Input: part model. Units: mm. Frame: model coordinates. Face numbers are marked on the shaded views. A direction names the side the tool comes from. Give positions to 0.01 mm unless a question says otherwise; leave off trailing zeros. Loops run counter-clockwise (first coordinate to the right, second up) from the corner with the lowest first, then second, coordinate; pieces in that order, holes last. Notation, with made-up numbers: (-17.5, 20.25) - (28.5, 20.25) arc R22 cw to (28.5, 39.25) - close; hole circle Ø2 at (68.25, -25). An arc over 180 degrees is marked (long way). Answer as a JSON object with one key per item and string values. Group by question number.
(1) Pin query (flat end, axial travel): P1, Ø2, axis at y = -14.5, z = 74, coming from the +X side; P2, Ø8, axis at x = -15.5, z = 73.5, coming from the -Y side; P3, Ø2, axis at x = 17, y = 10.5, coming from the -Z side (3 decimals). Return the tip coordinate at first contact, or that it passes through.
(2) Section query D-D (x = 18). Return loops of the section in (y, z) (3 decimals), plus the area to 3 significant figures.
(3) Section query B-B (y = 0). Return loops of the section in (x, z) (3 decimals), plus the area to 3 significant figures.
(4) Mould query, pull axis Y, two halves, no side actions, for the marked faces 1, 2, 3 and 4. Classes: +Y half, -Y half, draft (parallel to the pull), parting line (faces both ways), or undercut.
(5) Section query C-C (z = 80.25). Return loops of the section in (x, y).
(6) Access query for the marked faces 5, 6 and 7. Directions: +Z, -Z, +X, -X, +Y, -Y. A direction counts if a zero-diameter tool reaches every point of the face in a straight line with its end or side. Return the directions, or none.
(7) Material intervals for L1, parallel to Y at x = -1.5, z = 80.1; L2, parallel to Z at x = 14.5, y = 7.5 (3 decimals); L3, parallel to X at y = 0.5, z = 70.25, sorted ascending.
(8) Section query A-A (z = 69.25). Return loops of the section in (x, y).
Autodesk Inventor part; units mm, degrees
ref_plane "YZ Plane" through (0, 0, 0) normal (1, 0, 0) x (0, 1, 0)
ref_plane "XZ Plane" through (0, 0, 0) normal (0, 1, 0) x (-1, 0, 0)
ref_plane "XY Plane" through (0, 0, 0) normal (0, 0, 1) x (1, 0, 0)
sketch "Эскиз1" plane through (0, 0, 0) normal (0, 0, 1) x (1, 0, 0)
  circle A0 centre (0, 0) radius 22.5
  dimension "d0" = 45
extrude "Выдавливание1" add sketch "Эскиз1" along normal blind 9.295
sketch "Эскиз2" plane through (0, 0, 9.295) normal (0, 0, 1) x (1, 0, 0)
  circle A0 centre (0, 0) radius 12.6
  dimension "d3" = 25.2
extrude "Выдавливание2" add sketch "Эскиз2" along normal blind 7.8
sketch "Эскиз3" plane through (0, 0, 9.295) normal (0, 0, 1) x (1, 0, 0)
  circle A0 centre (0, 0) radius 12.6
  circle A1 centre (0, 0) radius 22.5
  circle A2 centre (0, 0) radius 14.6
  dimension "d6" = 2
extrude "Выдавливание3" add sketch "Эскиз3" along normal blind 1 contours A2
chamfer "Фаска1" distance 0.5 angle 45 1 edges at (-14.6, 0, 10.295)
sketch "Эскиз4" plane through (0, 0, 17.095) normal (0, 0, 1) x (1, 0, 0)
  line L0 (0, 0) -> (0, 4)
  line L1 (0, 4) -> (3.4641, 2)
  line L2 (3.4641, 2) -> (3.4641, -2)
  line L3 (3.4641, -2) -> (0, -4)
  line L4 (0, -4) -> (-3.4641, -2)
  line L5 (-3.4641, -2) -> (-3.4641, 2)
  line L6 (-3.4641, 2) -> (0, 4)
  line L7 (3.9641, 2.2887) -> (0, 4.5774)
  line L8 (0, 4.5774) -> (-3.9641, 2.2887)
  line L9 (-3.9641, 2.2887) -> (-3.9641, -2.2887)
  line L10 (-3.9641, -2.2887) -> (0, -4.5774)
  line L11 (0, -4.5774) -> (3.9641, -2.2887)
  line L12 (3.9641, -2.2887) -> (3.9641, 2.2887)
  dimension "d12" = 4
  dimension "d13" = 0.5
extrude "Выдавливание4" cut sketch "Эскиз4" against normal blind 7.8 contours L1 L2 L3 L4 L5 L6 | L12 L11 L10 L9 L8 L7
sketch "Эскиз5" plane through (0, 0, 0) normal (0, 0, -1) x (-1, 0, 0)
  circle A0 centre (13.4441, 11.2809) radius 1.5
  circle A1 centre (0, 17.55) radius 1.5
  circle A2 centre (-13.4441, 11.2809) radius 1.5
  circle A3 centre (13.4441, 11.2809) radius 2.1
  circle A4 centre (0, 17.55) radius 2.1
  circle A5 centre (-13.4441, 11.2809) radius 2.1
  point P0 (0, 0)
  dimension "d16" = 4.2
  dimension "d17" = 4.2
  dimension "d18" = 4.2
extrude "Выдавливание5" cut sketch "Эскиз5" against normal blind 7.8 contours A0 | A1 | A2 | A3 | A4 | A5
sketch "Эскиз6" plane through (0, 0, 17.095) normal (0, 0, 1) x (1, 0, 0)
  circle A0 centre (-1.5, -4.5) radius 1.5
  circle A1 centre (-1.5, -4.5) radius 3.5
  point P0 (0, 0)
  dimension "d21" = 7
extrude "Выдавливание6" cut sketch "Эскиз6" against normal blind 13 contours A0 | A1
sketch "Эскиз7" plane through (-1.5, -4.5, 4.095) normal (0, 0, 1) x (1, 0, 0)
  circle A0 centre (0, 0) radius 3.5
  circle A1 centre (0, 0) radius 1.6
  point P0 (1.5, 4.5)
  dimension "d24" = 3.2
extrude "Выдавливание7" cut sketch "Эскиз7" against normal blind 13 contours A1
ref_plane "РабПлоскость1" through (0, 0, 41.595) normal (0, 0, 1) x (1, 0, 0)
mirror "Зеркальное отражение1" about plane through (0, 0, 41.595) normal (0, 0, 1)
sketch "Эскиз8" plane through (0, 0, 0) normal (0, 0, -1) x (-1, 0, 0)
  circle A0 centre (0, 0) radius 38.8283
extrude "Выдавливание8" cut sketch "Эскиз8" against normal blind 20
properties part number "wheel_fixator_mirror"
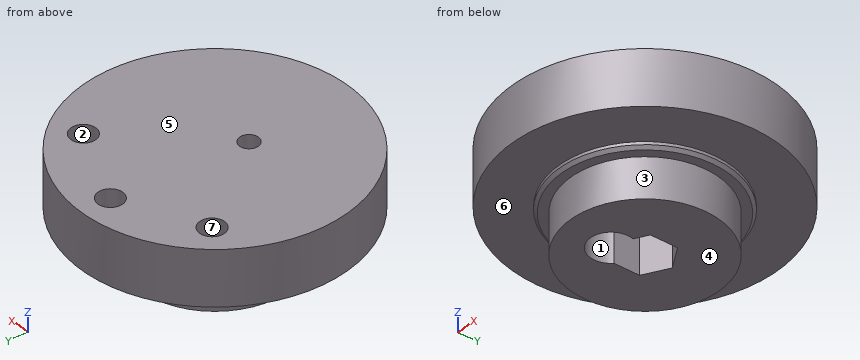
Recorded:
{
 "1": {"P1": "stops at x = 18", "P2": "stops at y = -19.33", "P3": "stops at z = 73.895"},
 "2": {"outline": "(-13.5, 73.895) - (13.5, 73.895) - (13.5, 83.19) - (-13.5, 83.19) - close", "area": "251 mm^2"},
 "3": {"outline": "(-22.5, 73.895) - (-14.6, 73.895) - (-14.6, 73.395) - (-14.1, 72.895) - (-12.6, 72.895) - (-12.6, 66.095) - (-3.964, 66.095) - (-3.964, 73.895) - (3.964, 73.895) - (3.964, 66.095) - (12.6, 66.095) - (12.6, 72.895) - (14.1, 72.895) - (14.6, 73.395) - (14.6, 73.895) - (22.5, 73.895) - (22.5, 83.19) - (-22.5, 83.19) - close", "area": "557 mm^2"},
 "4": {"face 1": "undercut", "face 2": "undercut", "face 3": "parting line", "face 4": "draft"},
 "5": {"outline": "circle Ø45 at (0, 0); hole circle Ø4.2 at (-13.44, 11.28); hole circle Ø3.2 at (-1.5, -4.5); hole circle Ø4.2 at (0, 17.55); hole circle Ø4.2 at (13.44, 11.28)"},
 "6": {"face 5": "+Z, +X, -X, +Y, -Y", "face 6": "-Z", "face 7": "+Z"},
 "7": {"L1": "y = -22.45 to -6.1, -2.9 to 16.08, 19.02 to 22.45", "L2": "z = 73.895 to 83.19", "L3": "x = -12.59 to -3.96, 3.96 to 12.59"},
 "8": {"outline": "circle Ø25.2 at (0, 0); hole (-3.96, -2.01) arc R3.5 ccw (long way) to (1.86, -3.51) - (3.96, -2.29) - (3.96, 2.29) - (0, 4.58) - (-3.96, 2.29) - close"}
}
